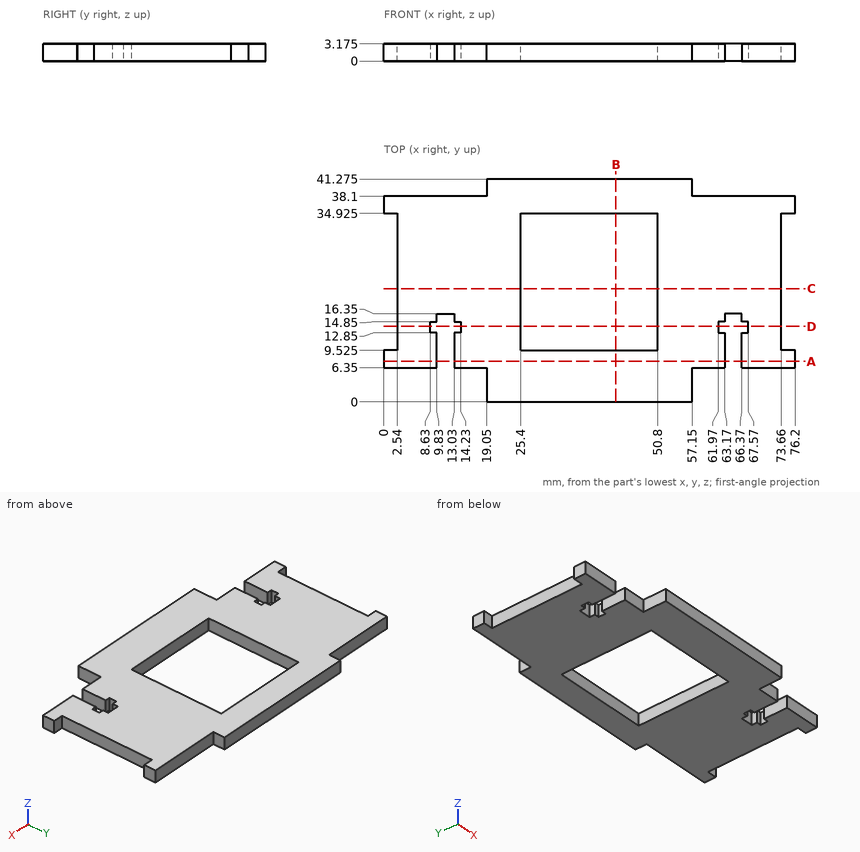
Geometry: see drawing. Coordinates: mm, zero at the bounding-box minimum. Coordinates: 2 decimals unless noted, no trailing zeros. Write each loop counter-clockwise with the first axis right and the second up, starting at its lowest first coordinate (ties: lowest second). Pieces come first, ordered by that corner, then holes. Notation, with made-up numbers: (68, 22) - (127, 22) arc R16 cw to (127, 33) - close; hole circle Ø6 at (-33, -13.5). An arc over 180 degrees is marked (long way). Put each result on its own line as item: value. Start each with the question number.
1) Cut plane C-C (y = 21). Return the cut outline in (x, z) (3 decimals), plus the area to 3 significant figures.
2) Cut plane D-D (y = 14). Return the cut outline in (x, z) (3 decimals).
3) Cut plane A-A (y = 7.5). Return the cut outline in (x, z) (3 decimals).
4) Contact query for flat-ended pins moving along their axis: pin 1 (1 mm diameter, centred on y = 39.5, z = 2, fed in from +X); pin 2 (1.3 mm diameter, centred on x = 13.5, z = 1, fed in from -Y); pin 3 (0.6 mm diameter, centred on x = 62.5, z = 1, fed in from +Y). Output: stop coordinate, or through.
5) Cut plane B-B (x = 43). Return the cut outline in (y, z) (3 decimals).
6) Ray query, L1, parallel to X at y = 15, z = 1.45; L2, parallel to X at y = 8, z = 0.45; L3, parallel to X at y = 28.5, z = 2.75. Return the intervals inside material, ascending.
Resolved:
1. outline: (2.54, 0) - (25.4, 0) - (25.4, 3.175) - (2.54, 3.175) - close; (50.8, 0) - (73.66, 0) - (73.66, 3.175) - (50.8, 3.175) - close
1. area: 145 mm2
2. outline: (2.54, 0) - (8.63, 0) - (8.63, 3.175) - (2.54, 3.175) - close; (14.23, 0) - (25.4, 0) - (25.4, 3.175) - (14.23, 3.175) - close; (50.8, 0) - (61.97, 0) - (61.97, 3.175) - (50.8, 3.175) - close; (67.57, 0) - (73.66, 0) - (73.66, 3.175) - (67.57, 3.175) - close
3. outline: (0, 0) - (9.83, 0) - (9.83, 3.175) - (0, 3.175) - close; (13.03, 0) - (63.17, 0) - (63.17, 3.175) - (13.03, 3.175) - close; (66.37, 0) - (76.2, 0) - (76.2, 3.175) - (66.37, 3.175) - close
4. pin 1: stops at x = 57.15
4. pin 2: stops at y = 6.35
4. pin 3: stops at y = 38.1
5. outline: (0, 0) - (9.525, 0) - (9.525, 3.175) - (0, 3.175) - close; (34.925, 0) - (41.275, 0) - (41.275, 3.175) - (34.925, 3.175) - close
6. L1: x = 2.54 to 9.83, 13.03 to 25.4, 50.8 to 63.17, 66.37 to 73.66
6. L2: x = 0 to 9.83, 13.03 to 63.17, 66.37 to 76.2
6. L3: x = 2.54 to 25.4, 50.8 to 73.66
